Geometry check sheet. Reference: the model listing, model coordinates, mm. Face numbers are marked on the shaded views. A direction names the side the tool comes from. Coordinates: 2 decimals unless noted, no trailing zeros. Write each loop counter-clockwise with the first axis right and the second up, starting at its lowest first coordinate (ties: lowest second). Pieces come first, ordered by that corner, then holes. Notation, with made-up numbers: (62.25, -28.5) -> (92.25, -28.5) arc R27 ccw to (92.25, -11.5) -> close; hole circle Ø9 at (7.25, 85.5). An arc over 180 degrees is marked (long way). Answer in a Markdown table with one row per item. Add a question column.
Q1. Section check C-C, the plane x = -127. Record the boundary of the cut face in (y, z), and give its area (3 significant figures).
Q2. Gauge pin test, flat ends, axial feed: P1, Ø0.6, axis at x = -149, z = 16, coming from the -Y side; P2, Ø7.5, axis at y = 37.23, z = 63.19, coming from the -X side; P3, Ø4.5, axis at x = -148.03, y = 44.95, coming from the -Z side; P4, Ø4.5, axis at x = -114.5, y = 44, coming from the -Z side. Record the tip position at first contact, or that the pin passes through.
Q3. Thickness scan on line 1 (X direction, y = 62, z = 13); line 2 (Z direction, x = -148, y = 75); line 3 (Z direction, x = -137.5, y = 59.5). Record the ranges inside material, lowest first.
Q4. Tool access check on the marked faces 4, 5, 6, 7 and 8. Record the directions out of +Z, -Z, +X, -X, +Y, -Y that give a thin tool (end or side, any length) a straight path to the whole face; none if there is none.
Q5. Section check B-B, the plane z = 5.5. Count the separate pieces of the cut face and the enclosed holes in it, and give its area (3 significant figures).
Q6. Section check D-D, the plane z = 53. Record the boundary of the cut face in (x, y).
Q7. Section check A-A, the plane y = 68. Record the boundary of the cut face in (x, z).
Q8. Release check for a two-part mould opening along Y. For the marked faces 1, 2 and 3 record: pulls with the +Y half, pulls with the -Y half, needs draft (parallel to the pull), parting line crosses it, or undercut.
```python
from build123d import *

# Parameters (mm, degrees)
CROQUIS2_R              = 2.5
SALIENTE_EXTRUIR1_DEPTH = 3
SALIENTE_EXTRUIR2_DEPTH = 40
CROQUIS4_R              = 2.5
SALIENTE_EXTRUIR3_DEPTH = 12
CROQUIS6_R              = 2.3
CROQUIS6_R_2            = 1
SALIENTE_EXTRUIR5_DEPTH = 4.000002
SALIENTE_EXTRUIR6_START = -36.000002
CROQUIS6_2_R            = 2.3
CROQUIS6_2_R_2          = 1
SALIENTE_EXTRUIR6_DEPTH = 3.999998
CROQUIS7_R              = 12
CORTAR_EXTRUIR1_DEPTH   = 3


with BuildPart() as part:
    # Croquis2 → Saliente-Extruir1 (new body)
    with BuildSketch(Plane.XY):
        with BuildLine():
            Line((-152.030771759, 47.953613054), (-152.030771759, 99.953613054))
            Line((-152.030771759, 99.953613054), (-112.030771759, 99.953613054))
            Line((-112.030771759, 99.953613054), (-112.030771759, 47.953613054))
            ThreePointArc((-112.030771759, 47.953613054), (-114.449632929, 40.210196563), (-121.030771759, 44.953613054))
            Line((-121.030771759, 44.953613054), (-143.030771759, 44.953613054))
            ThreePointArc((-143.030771759, 44.953613054), (-149.611910589, 40.210196563), (-152.030771759, 47.953613054))
        make_face()
        with Locations((-148.030771759, 44.953613054)):
            Circle(CROQUIS2_R, mode=Mode.SUBTRACT)
        with Locations((-116.030771759, 44.953613054)):
            Circle(CROQUIS2_R, mode=Mode.SUBTRACT)
    extrude(amount=SALIENTE_EXTRUIR1_DEPTH)

    # Croquis3 → Saliente-Extruir2 (add)
    with BuildSketch(Plane.ZY.offset(152.030771759)):
        Polygon((3, 99.953613054), (16.75, 99.953613054), (55.851046981, 77.378613054), (42.101046981, 53.56291445), (3, 76.13791445), align=None)
        Polygon((15.25, 97.355536842), (4.5, 78.735990661), (41.00297077, 57.660990661), (51.75297077, 76.280536842), align=None, mode=Mode.SUBTRACT)
    extrude(amount=-SALIENTE_EXTRUIR2_DEPTH)

    # Croquis4 → Saliente-Extruir3 (add)
    # profile 1 of 2: a face of its own
    with BuildSketch(Plane.XY.offset(3)):
        with BuildLine():
            Line((-152.030771759, 47.953613054), (-152.030771759, 49.953613054))
            Line((-152.030771759, 49.953613054), (-148.030771759, 49.953613054))
            ThreePointArc((-148.030771759, 49.953613054), (-145.794703781, 40.481477099), (-152.030771759, 47.953613054))
        make_face()
        with Locations((-148.030771759, 44.953613054)):
            Circle(CROQUIS4_R, mode=Mode.SUBTRACT)
    # profile 2 of 2: a face of its own
    with BuildSketch(Plane.XY.offset(3)):
        with BuildLine():
            Line((-112.030771759, 49.953613054), (-112.030771759, 47.953613054))
            ThreePointArc((-112.030771759, 47.953613054), (-118.266839736, 40.481477099), (-116.030771759, 49.953613054))
            Line((-116.030771759, 49.953613054), (-112.030771759, 49.953613054))
        make_face()
        with Locations((-116.030771759, 44.953613054)):
            Circle(CROQUIS4_R, mode=Mode.SUBTRACT)
    extrude(amount=SALIENTE_EXTRUIR3_DEPTH)

    # Croquis6 → Saliente-Extruir5 (add)
    with BuildSketch(Plane.ZY.offset(152.030771759)):
        with BuildLine():
            Line((3, 49.953613054), (3, 76.13791445))
            Line((3, 76.13791445), (66.916006899, 39.235990661))
            ThreePointArc((66.916006899, 39.235990661), (68.313784378, 35.861457314), (65.416006899, 33.63791445))
            Line((65.416006899, 33.63791445), (17, 33.63791445))
            Line((17, 33.63791445), (17, 49.953613054))
            Line((17, 49.953613054), (3, 49.953613054))
        make_face()
        with Locations((63.194377499, 37.233198253)):
            Circle(CROQUIS6_R, mode=Mode.SUBTRACT)
        with Locations((48.705490104, 41.11548393)):
            Circle(CROQUIS6_R_2, mode=Mode.SUBTRACT)
    extrude(amount=-SALIENTE_EXTRUIR5_DEPTH)

    # Croquis6<2> → Saliente-Extruir6 (add)
    with BuildSketch(Plane.ZY.offset(152.030771759).offset(SALIENTE_EXTRUIR6_START)):
        with BuildLine():
            Line((3, 49.953613054), (3, 76.13791445))
            Line((3, 76.13791445), (66.916006899, 39.235990661))
            ThreePointArc((66.916006899, 39.235990661), (68.313784378, 35.861457314), (65.416006899, 33.63791445))
            Line((65.416006899, 33.63791445), (17, 33.63791445))
            Line((17, 33.63791445), (17, 49.953613054))
            Line((17, 49.953613054), (3, 49.953613054))
        make_face()
        with Locations((63.194377499, 37.233198253)):
            Circle(CROQUIS6_2_R, mode=Mode.SUBTRACT)
        with Locations((48.705490104, 41.11548393)):
            Circle(CROQUIS6_2_R_2, mode=Mode.SUBTRACT)
    extrude(amount=-SALIENTE_EXTRUIR6_DEPTH)

    # Croquis7 → Cortar-Extruir1 (cut)
    with BuildSketch(Plane(origin=(0, 82.218172547, 47.468684052), x_dir=(1, 0, 0), z_dir=(0, 0.8660254037844388, 0.49999999999999983))):
        with Locations((-149.530771759, 12.895881013)):
            Circle(CROQUIS7_R)
    extrude(amount=-CORTAR_EXTRUIR1_DEPTH, mode=Mode.SUBTRACT)


solid = part.part
```
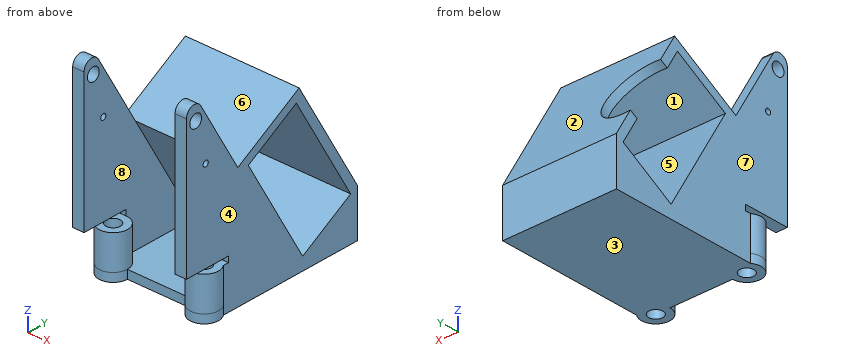
Calculated:
| question | item | result |
|---|---|---|
| 1 | outline | (44.95, 0) -> (99.95, 0) -> (99.95, 16.75) -> (77.38, 55.85) -> (53.56, 42.1) -> (76.14, 3) -> (44.95, 3) -> close; hole (57.66, 41) -> (78.74, 4.5) -> (97.36, 15.25) -> (76.28, 51.75) -> close |
| 1 | area | 664 mm² |
| 2 | P1 | stops at y = 49.95 |
| 2 | P2 | stops at x = -152.03 |
| 2 | P3 | stops at z = 17 |
| 2 | P4 | stops at z = 0 |
| 3 | line 1 | x = -152.03 to -148.03, -116.03 to -112.03 |
| 3 | line 2 | z = 0 to 3, 4.97 to 10.97, 51.01 to 54.48 |
| 3 | line 3 | z = 0 to 3, 31.82 to 37.82, 42.06 to 45.53 |
| 4 | face 4 | +Z, +X, +Y |
| 4 | face 5 | +X, -X |
| 4 | face 6 | +Z, +X, -X |
| 4 | face 7 | +Z, -X, +Y |
| 4 | face 8 | none |
| 5 | separate pieces | 2 |
| 5 | enclosed holes | 2 |
| 5 | area | 1,240 mm² |
| 6 | outline | (-152.03, 33.64) -> (-148.03, 33.64) -> (-148.03, 47.27) -> (-152.03, 47.27) -> close; (-152.03, 72.44) -> (-112.03, 72.44) -> (-112.03, 79.02) -> (-152.03, 79.02) -> close; (-116.03, 33.64) -> (-112.03, 33.64) -> (-112.03, 47.27) -> (-116.03, 47.27) -> close |
| 7 | outline | (-152.03, 0) -> (-112.03, 0) -> (-112.03, 23.1) -> (-152.03, 23.1) -> close; (-152.03, 46.97) -> (-112.03, 46.97) -> (-112.03, 50.44) -> (-152.03, 50.44) -> close; hole (-148.03, 3) -> (-116.03, 3) -> (-116.03, 17.1) -> (-148.03, 17.1) -> close |
| 8 | face 1 | undercut |
| 8 | face 2 | pulls with the +Y half |
| 8 | face 3 | needs draft |
